from build123d import *

# Parameters (mm, degrees)
SKETCH1_W           = 82
SKETCH1_H           = 85
BOSS_EXTRUDE1_DEPTH = 1.2
SKETCH2_W           = 60
SKETCH2_H           = 30
CUT_EXTRUDE1_DEPTH  = 2
SKETCH3_W           = 60
SKETCH3_H           = 15
CUT_EXTRUDE2_DEPTH  = 2
SKETCH4_W           = 82
SKETCH4_H           = 85
SKETCH4_W_2         = 79.6
SKETCH4_H_2         = 82.6
BOSS_EXTRUDE2_DEPTH = 20
SKETCH5_W           = 62.4
SKETCH5_H           = 17.4
SKETCH5_W_2         = 60
SKETCH5_H_2         = 15
BOSS_EXTRUDE4_DEPTH = 20
SKETCH10_W          = 1.2
SKETCH10_H          = 3.8
BOSS_EXTRUDE5_DEPTH = 20
SKETCH11_W          = 5
SKETCH11_H          = 11.2
CUT_EXTRUDE3_DEPTH  = 1.5
SKETCH12_W          = 21.5
SKETCH12_H          = 8
CUT_EXTRUDE4_DEPTH  = 1.5
SKETCH15_W          = 20.5
SKETCH15_H          = 5
CUT_EXTRUDE5_DEPTH  = 1.5


with BuildPart() as part:
    # Sketch1 → Boss-Extrude1 (new body)
    with BuildSketch(Plane(origin=(0, 0, 0), x_dir=(1, 0, 0), z_dir=(0, 1, 0))):
        with Locations((41, 42.5)):
            Rectangle(SKETCH1_W, SKETCH1_H)
    extrude(amount=BOSS_EXTRUDE1_DEPTH)

    # Sketch2 → Cut-Extrude1 (cut)
    with BuildSketch(Plane(origin=(0, 1.2, 0), x_dir=(1, 0, 0), z_dir=(0, 1, 0))):
        with Locations((41, 64.7)):
            Rectangle(SKETCH2_W, SKETCH2_H)
    extrude(amount=-CUT_EXTRUDE1_DEPTH, mode=Mode.SUBTRACT)

    # Sketch3 → Cut-Extrude2 (cut)
    with BuildSketch(Plane(origin=(0, 1.2, 0), x_dir=(1, 0, 0), z_dir=(0, 1, 0))):
        with Locations((41, 37.5)):
            Rectangle(SKETCH3_W, SKETCH3_H)
    extrude(amount=-CUT_EXTRUDE2_DEPTH, mode=Mode.SUBTRACT)

    # Sketch4 → Boss-Extrude2 (add)
    with BuildSketch(Plane.XZ):
        with Locations((41, -42.5)):
            Rectangle(SKETCH4_W, SKETCH4_H)
        with Locations((41, -42.5)):
            Rectangle(SKETCH4_W_2, SKETCH4_H_2, mode=Mode.SUBTRACT)
    extrude(amount=BOSS_EXTRUDE2_DEPTH)

    # Sketch5 → Boss-Extrude4 (add)
    with BuildSketch(Plane.XZ):
        with Locations((41, -37.5)):
            Rectangle(SKETCH5_W, SKETCH5_H)
        with Locations((41, -37.5)):
            Rectangle(SKETCH5_W_2, SKETCH5_H_2, mode=Mode.SUBTRACT)
    extrude(amount=BOSS_EXTRUDE4_DEPTH)

    # Sketch10 → Boss-Extrude5 (add)
    with BuildSketch(Plane.XZ):
        with Locations((9.8, -26.9)):
            Rectangle(SKETCH10_W, SKETCH10_H)
    extrude(amount=BOSS_EXTRUDE5_DEPTH)

    # Sketch11 → Cut-Extrude3 (cut)
    with BuildSketch(Plane.ZY):
        with Locations((-24.5, -9.4)):
            Rectangle(SKETCH11_W, SKETCH11_H)
    extrude(amount=-CUT_EXTRUDE3_DEPTH, mode=Mode.SUBTRACT)

    # Sketch12 → Cut-Extrude4 (cut)
    with BuildSketch(Plane(origin=(0, 0, -85), x_dir=(-1, 0, 0), z_dir=(0, 0, -1))):
        with Locations((-57.4, -4.3)):
            Rectangle(SKETCH12_W, SKETCH12_H)
    extrude(amount=-CUT_EXTRUDE4_DEPTH, mode=Mode.SUBTRACT)

    # Sketch15 → Cut-Extrude5 (cut)
    with BuildSketch(Plane.XY.offset(-45)):
        with Locations((58.25, -2.8)):
            Rectangle(SKETCH15_W, SKETCH15_H)
    extrude(amount=-CUT_EXTRUDE5_DEPTH, mode=Mode.SUBTRACT)


solid = part.part
Work out the finished part from the listing and answer in its coordinate system (mm). A direction names the side the tool comes from. Round coordinates to 2 decimals unless told otherwise and drop trailing zeros. Write each loop counter-clockwise with the first axis right and the second up, starting at its lowest first coordinate (ties: lowest second). Pieces come first, ordered by that corner, then holes. Notation, with made-up numbers: (80.25, 9.25) - (113.25, 9.25) arc R26 ccw to (113.25, 38.25) - close; hole circle Ø4 at (11, 15). An arc over 180 degrees is marked (long way). Answer in a Markdown table with one row per item. Add a question column.
1. Find the intervals of material crossed by line 1 along Z through (x, y) = (24.5, -4); line 2 along Z through (x, y) = (63, -2); line 3 along X through (y, z) = (-7, -72), in increasing order. Write a range as from..to.
2. A cutting plane is placed at D-D, the plane z = -68. Determine the outline of the cut face in (x, y).
3. A cutting plane is placed at C-C, the plane y = -10.75. Determine the outline of the cut face in (x, z), and give its area (3 significant figures).
4. For faces 1 (the flat face through (71, -9, -38)), 2 (the flat face through (82, -9, -43)), 3 (the flat face through (10.4, -10, -27)), determine the directions among +Z, -Z, +X, -X, +Y, -Y from which every point of the face is accessible in a straight line to the end or side of a thin tool.
5. The mould has two halves that part along Z. Classify faces 4 (the flat face through (0, -9, -43)), 5 (the flat face through (40, -10, -1.2)), 6 (the flat face through (40, -9, -85)): +Z half, -Z half, draft (parallel to the pull), parting line (faces both ways), or undercut.
6. A cutting plane is placed at A-A, the plane y = -16.25. Determine the outline of the cut face in (x, z), and give its area (3 significant figures).
7. A cutting plane is placed at B-B, the plane x = 34. Determine the outline of the cut face in (y, z).
Worked out:
| question | item | result |
|---|---|---|
| 1 | line 1 | -85..-83.8, -46.2..-45, -30..-28.8, -1.2..0 |
| 1 | line 2 | -30..-28.8, -1.2..0 |
| 1 | line 3 | 0..1.2, 80.8..82 |
| 2 | outline | (0, -20) - (1.2, -20) - (1.2, 0) - (11, 0) - (11, 1.2) - (0, 1.2) - close; (71, 0) - (80.8, 0) - (80.8, -20) - (82, -20) - (82, 1.2) - (71, 1.2) - close |
| 3 | outline | (0, -85) - (82, -85) - (82, 0) - (0, 0) - (0, -22) - (1.2, -22) - (1.2, -1.2) - (80.8, -1.2) - (80.8, -83.8) - (1.2, -83.8) - (1.2, -27) - (0, -27) - close; (9.2, -28.8) - (9.8, -28.8) - (9.8, -46.2) - (72.2, -46.2) - (72.2, -28.8) - (10.4, -28.8) - (10.4, -25) - (9.2, -25) - close; hole (11, -45) - (71, -45) - (71, -30) - (11, -30) - close |
| 3 | area | 579 mm^2 |
| 4 | face 1 | +Y, -Y |
| 4 | face 2 | +Z, -Z, +X, +Y, -Y |
| 4 | face 3 | -Y |
| 5 | face 4 | draft |
| 5 | face 5 | undercut |
| 5 | face 6 | -Z half |
| 6 | outline | (0, -85) - (82, -85) - (82, 0) - (0, 0) - close; (9.2, -28.8) - (9.8, -28.8) - (9.8, -46.2) - (72.2, -46.2) - (72.2, -28.8) - (10.4, -28.8) - (10.4, -25) - (9.2, -25) - close; hole (1.2, -83.8) - (80.8, -83.8) - (80.8, -1.2) - (1.2, -1.2) - close; hole (11, -45) - (71, -45) - (71, -30) - (11, -30) - close |
| 6 | area | 585 mm^2 |
| 7 | outline | (-20, -85) - (1.2, -85) - (1.2, -79.7) - (0, -79.7) - (0, -83.8) - (-20, -83.8) - close; (-20, -46.2) - (0, -46.2) - (0, -49.7) - (1.2, -49.7) - (1.2, -45) - (-20, -45) - close; (-20, -30) - (1.2, -30) - (1.2, 0) - (-20, 0) - (-20, -1.2) - (0, -1.2) - (0, -28.8) - (-20, -28.8) - close |
